from build123d import *

# Parameters (mm, degrees)
PAD_DEPTH         = 5
POCKET_DEPTH      = 5.001
POCKET_DEPTH_BACK = -5.001


with BuildPart() as part:
    # Sketch → Pad (new body, symmetric)
    with BuildSketch(Plane.XY):
        Polygon((-5, 4), (-2.45, 4), (-2.45, 7.6), (-5, 7.6), (-5, 11.6), (5, 11.6), (5, 7.6), (2.45, 7.6), (2.45, 4), (5, 4), (5, 2.5), (2.5, 0), (-2.5, 0), (-5, 2.5), align=None)
    extrude(amount=PAD_DEPTH, both=True)

    # Sketch001 → Pocket (cut, two sides)
    with BuildSketch(Plane.YZ) as pocket_sk:
        Polygon((11.6, 2.5), (11.6, -2.5), (9.1, -5), (7.6, -5), (7.6, -2.45), (4, -2.45), (4, -6.892367), (13.16095, -6.892367), (13.16095, 6.892367), (4, 6.892367), (4, 2.45), (7.6, 2.45), (7.6, 5), (9.1, 5), align=None)
    extrude(amount=-POCKET_DEPTH, mode=Mode.SUBTRACT)
    extrude(pocket_sk.sketch, amount=-POCKET_DEPTH_BACK, mode=Mode.SUBTRACT)


solid = part.part
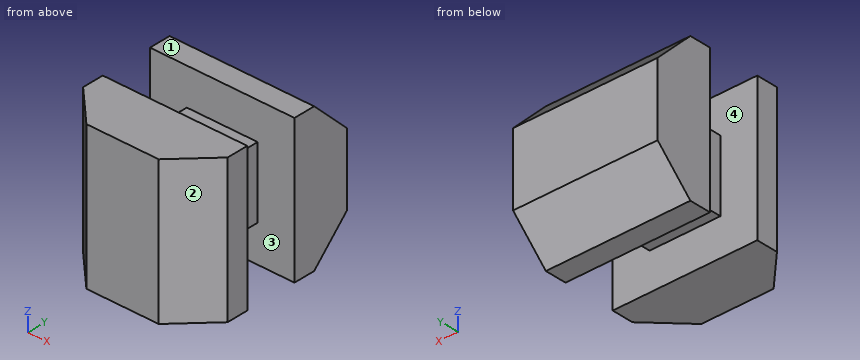
Build history of the part. All positions in model axes, mm. Face numbers are marked on the shaded views. Give positions to 0.01 mm unless a question says otherwise; leave off trailing zeros. Loops run counter-clockwise (first coordinate to the right, second up) from the corner with the lowest first, then second, coordinate; pieces in that order, holes last. Notation, with made-up numbers: (6.5, 43) -> (47.5, 43) arc R35 cw to (47.5, 75) -> close; hole circle Ø3 at (-29.5, 74.5). An arc over 180 degrees is marked (long way). Answer in a Markdown table with one row per item.
Item 1: Probe line 1 along X through (y, z) = (6.75, -1.75); line 2 along Y through (x, z) = (3.5, 0.5); line 3 along Y through (x, z) = (2, -3). List the from-to ranges inside material, lowest first. Write a range as [from, to].
Findings below:
| item | result |
|---|---|
| line 1 | x = [-2.45, 2.45] |
| line 2 | y = [1, 4], [7.6, 11.6] |
| line 3 | y = [0, 4], [7.6, 11.1] |
Item 2: Slice it at D-D on x = 1.5. Write the cut outline in (y, z).
Findings below:
| item | result |
|---|---|
| outline | (0, -5) -> (4, -5) -> (4, -2.45) -> (7.6, -2.45) -> (7.6, -5) -> (9.1, -5) -> (11.6, -2.5) -> (11.6, 2.5) -> (9.1, 5) -> (7.6, 5) -> (7.6, 2.45) -> (4, 2.45) -> (4, 5) -> (0, 5) -> close |
Item 3: Slice it at B-B on x = -2.75. Write the cut outline in (y, z), plus the area to 4 significant figures.
Findings below:
| item | result |
|---|---|
| outline | (0.25, -5) -> (4, -5) -> (4, 5) -> (0.25, 5) -> close; (7.6, -5) -> (9.1, -5) -> (11.6, -2.5) -> (11.6, 2.5) -> (9.1, 5) -> (7.6, 5) -> close |
| area | 71.25 mm² |
Item 4: Slice it at C-C on z = 0. Write the cut outline in (x, y).
Findings below:
| item | result |
|---|---|
| outline | (-5, 2.5) -> (-2.5, 0) -> (2.5, 0) -> (5, 2.5) -> (5, 4) -> (2.45, 4) -> (2.45, 7.6) -> (5, 7.6) -> (5, 11.6) -> (-5, 11.6) -> (-5, 7.6) -> (-2.45, 7.6) -> (-2.45, 4) -> (-5, 4) -> close |
Item 5: Flat gauge pins, fed straight in: P1, Ø1.1, axis at y = 6, z = 0.5, coming from the -X side; P2, Ø4, axis at x = -0.5, y = 5.5, coming from the -Z side; P3, Ø1.1, axis at x = 0, y = 6.5, coming from the +Z side; P4, Ø1.8, axis at y = 6.5, z = 0.5, coming from the +X side. Where does each tip first touch, or does it go through?
Findings below:
| item | result |
|---|---|
| P1 | stops at x = -2.45 |
| P2 | stops at z = -5 |
| P3 | stops at z = 2.45 |
| P4 | stops at x = 2.45 |
Item 6: Slice it at A-A on z = -4. Write the cut outline in (x, y).
Findings below:
| item | result |
|---|---|
| outline | (-5, 2.5) -> (-2.5, 0) -> (2.5, 0) -> (5, 2.5) -> (5, 4) -> (-5, 4) -> close; (-5, 7.6) -> (5, 7.6) -> (5, 10.1) -> (-5, 10.1) -> close |
Item 7: Mould opens along Y. For the marked faces 1, 2, 3 and 4 say: pulls with the +Y half, pulls with the -Y half, needs draft (parallel to the pull), parting line crosses it, or undercut.
Findings below:
| item | result |
|---|---|
| face 1 | needs draft |
| face 2 | pulls with the -Y half |
| face 3 | undercut |
| face 4 | undercut |
